```python
from build123d import *

# Parameters (mm, degrees)
ESQUISSE1_R        = 6.35
BOSS_EXTRU_1_DEPTH = 25.4
BOSS_EXTRU_2_DEPTH = 6.35


with BuildPart() as part:
    # Esquisse1 → Boss.-Extru.1 (new body)
    with BuildSketch(Plane.XY):
        Circle(ESQUISSE1_R)
    extrude(amount=BOSS_EXTRU_1_DEPTH)

    # Esquisse2 → Boss.-Extru.2 (add)
    with BuildSketch(Plane.XY.offset(25.4)):
        Polygon((9.525, 3.945384182), (3.945384182, 9.525), (-3.945384182, 9.525), (-9.525, 3.945384182), (-9.525, -3.945384182), (-3.945384182, -9.525), (3.945384182, -9.525), (9.525, -3.945384182), align=None)
    extrude(amount=BOSS_EXTRU_2_DEPTH)


solid = part.part
```
CAD build for the part. Positions are in the model's coordinates, mm. A direction names the side the tool comes from. Give positions to 0.01 mm unless a question says otherwise; leave off trailing zeros. Write each loop counter-clockwise with the first axis right and the second up, starting at its lowest first coordinate (ties: lowest second). Pieces come first, ordered by that corner, then holes. Notation, with made-up numbers: M 23.5,-12 L 67.5,-12 A28 cw 67.5,15 Z; hole C 7,23 d3. An arc over 180 degrees is marked long. Return JSON: item names as keys, results as strings. Group by question number.
(1) Drill centre lines: L1, parallel to Z at x = 2.25, y = 8.25; L2, parallel to X at y = 0.25, z = 24.5. Where is each one in solid material? Low to high. Write a range as [from, to].
(2) 3-axis set-ups, long thin cutter, end or side, ignore diameter. For faces 1 (the face through (-1.38, -6.2, 12.52)), 2 (the face through (6.77, 6.7, 28.53)): which of +Z, -Z, +X, -X, +Y, -Y reach the whole face in a straight line?
(3) Band-saw the part on C-C (z = 23). Give the cut face in (x, y).
(4) Band-saw the part on D-D (y = 7). Give the cut face in (x, z).
(5) Band-saw the part on B-B (x = 0). Give the cut face in (y, z) (3 decimals).
(6) Flat gauge pins, fed straight in: pin 1 Ø1.5 at (x, z) = (4.5, 10.5) entering from +Y; pin 2 Ø4 at (x, z) = (0.5, 13.5) entering from +Y; pin 3 Ø1.5 at (y, z) = (2.5, 17) entering from +X. Where does each tip first touch, or does it go through?
(7) Band-saw the part on A-A (z = 27). Give the cut face in (x, y) (3 decimals), and give its area (3 significant figures).
Entries:
{
 "1": {"L1": "z = [25.4, 31.75]", "L2": "x = [-6.35, 6.35]"},
 "2": {"face 1": "-Z", "face 2": "+Z, -Z, +X, +Y"},
 "3": {"outline": "C 0,0 d12.7"},
 "4": {"outline": "M -6.47,25.4 L 6.47,25.4 L 6.47,31.75 L -6.47,31.75 Z"},
 "5": {"outline": "M -9.525,25.4 L -6.35,25.4 L -6.35,0 L 6.35,0 L 6.35,25.4 L 9.525,25.4 L 9.525,31.75 L -9.525,31.75 Z"},
 "6": {"pin 1": "stops at y = 5.12", "pin 2": "stops at y = 6.35", "pin 3": "stops at x = 6.1"},
 "7": {"outline": "M -9.525,-3.945 L -3.945,-9.525 L 3.945,-9.525 L 9.525,-3.945 L 9.525,3.945 L 3.945,9.525 L -3.945,9.525 L -9.525,3.945 Z", "area": "301 mm^2"}
}
